Check sheet for the modelled part. Datum: model origin and axes. Units: mm. A direction names the side the tool comes from. Round coordinates to 2 decimals unless told otherwise and drop trailing zeros. Write each loop counter-clockwise with the first axis right and the second up, starting at its lowest first coordinate (ties: lowest second). Pieces come first, ordered by that corner, then holes.
Item 1: Cross-section at B-B on x = 10.75. Enter the section's corners in (y, z).
Item 2: Release check for a two-part mould opening along Y. For faces 4 (the flat face through (11, -1, 1.8)), 5 (the flat face through (0, 0, 0)), 6 (the flat face through (2, -8, 0)) record: +Y half, -Y half, draft (parallel to the pull), parting line (faces both ways), or undercut.
Item 3: Material ranges on line 1 (Y direction, x = 11.25, z = 0.2); line 2 (Y direction, x = -3, z = -0.7); line 3 (Y direction, x = 7, z = 0.6), recorded low to high.
Item 4: Tool access check on faces 1 (the flat face through (8.8, -3.3, -0.2)), 2 (the flat face through (4, -7, 1.8)), 3 (the flat face through (9, 1, 1)). Record the directions out of +Z, -Z, +X, -X, +Y, -Y that give a thin tool (end or side, any length) a straight path to the whole face; none if there is none.
Item 5: Cross-section at D-D on x = -3. Enter the section's corners in (y, z), plus the area to 4 significant figures.
Item 6: Cross-section at A-A on z = 0.8. Enter the section's corners in (x, y), plus the area to 3 significant figures.
Item 7: Cross-section at C-C on y = 0. Enter the section's corners in (x, z).
Item 8: Go/stop test with flat-tipped pins: pin 1 Ø0.5 at (y, z) = (3, -1) entering from +X; pin 2 Ø0.5 at (y, z) = (4.5, 1) entering from -X; pin 3 Ø1.5 at (x, y) = (0.5, 2) entering from +Z. Record where each tip stops, or that it passes through.
Autodesk Fusion 360 part; units mm, degrees
sketch "Main Body" plane through (0, 0, 0) normal (0, 0, 1) x (1, 0, 0)
  line L0 (9, 8) -> (-9, 8)
  line L1 (-9, 8) -> (-9, -8)
  line L2 (-9, -8) -> (9, -8)
  line L3 (9, -8) -> (9, 8)
  line L4 (9, 8) -> (-9, -8) construction
  line L5 (-9, 8) -> (9, -8) construction
  line L6 (9, 8) -> (13, 8)
  line L7 (13, 8) -> (13, -8)
  line L8 (13, -8) -> (9, -8)
  line L9 (9, -8) -> (9, 8)
  line L10 (9, 6) -> (-9, 6)
  line L11 (-9, -6) -> (9, -6)
  line L12 (2, 3.3) -> (13, 3.3)
  line L13 (13, 3.3) -> (13, 2.7)
  line L14 (13, 2.7) -> (2, 2.7)
  line L15 (2, 2.7) -> (2, 3.3)
  circle A0 centre (-3, 0) radius 0.85
  point P0 (2, 3)
  dimension "d4" = 18
  dimension "d5" = 4
  dimension "d7" = 16
  dimension "d8" = -2
  dimension "d9" = -2
  dimension "d10" = 0.6
  dimension "d11" = 7
  dimension "d12" = 3
  dimension "d26" = 1.7
  dimension "d27" = 6
extrude "Base" add sketch "Main Body" against normal blind 1.5 contours L0 L1 L3 L9 L10 | L3 L6 L7 L9 L12 | L1 L3 L9 L10 L11 L12 L14 L15 | L3 L7 L9 L12 L13 L14 | L3 L9 L12 L14 L15 | L1 L2 L3 L9 L11 | L3 L7 L8 L9 L14 | A0
extrude "Guide" add sketch "Main Body" along normal blind 1.8 contours L0 L1 L3 L9 L10 | L3 L6 L7 L9 L12 | L3 L7 L9 L12 L13 L14 | L1 L2 L3 L9 L11 | L3 L7 L8 L9 L14
extrude "Bristle Cut" cut sketch "Main Body" along normal through all and the other way through all contours L3 L7 L9 L12 L13 L14 | L3 L9 L12 L14 L15
pattern_linear "Bristle Pattern" count 3 spacing 3 along (0, -1, 0) of "Bristle Cut"
extrude "Fixing Hole" cut sketch "Main Body" against normal through all contours A0
equation "SegmentLength = 18 mm"
equation "d4 = SegmentLength"
equation "BandWidth = 12 mm"
equation "d7 = BandWidth + 4 mm"
equation "d11 = SegmentLength - 11 mm"
equation "d12 = BandWidth / NumBristles"
equation "d15 = BandThickness - 0.2 mm"
equation "d19 = NumBristles - 1"
equation "BandThickness = 2 mm"
Response values:
1. outline: (-8, -1.5) - (-3.3, -1.5) - (-3.3, 1.8) - (-8, 1.8) - close; (-2.7, -1.5) - (-0.3, -1.5) - (-0.3, 1.8) - (-2.7, 1.8) - close; (0.3, -1.5) - (2.7, -1.5) - (2.7, 1.8) - (0.3, 1.8) - close; (3.3, -1.5) - (8, -1.5) - (8, 1.8) - (3.3, 1.8) - close
2. face 4: draft
2. face 5: undercut
2. face 6: -Y half
3. line 1: y = -8 to -3.3, -2.7 to -0.3, 0.3 to 2.7, 3.3 to 8
3. line 2: y = -8 to -0.85, 0.85 to 8
3. line 3: y = -8 to -6, 6 to 8
4. face 1: +Z, -Z, +X
4. face 2: +Z, +X, -X, +Y, -Y
4. face 3: +Z, -X
5. outline: (-8, -1.5) - (-0.85, -1.5) - (-0.85, 0) - (-6, 0) - (-6, 1.8) - (-8, 1.8) - close; (0.85, -1.5) - (8, -1.5) - (8, 1.8) - (6, 1.8) - (6, 0) - (0.85, 0) - close
5. area: 28.65 mm2
6. outline: (-9, -8) - (13, -8) - (13, -3.3) - (9, -3.3) - (9, -6) - (-9, -6) - close; (-9, 6) - (9, 6) - (9, 3.3) - (13, 3.3) - (13, 8) - (-9, 8) - close; (9, -2.7) - (13, -2.7) - (13, -0.3) - (9, -0.3) - close; (9, 0.3) - (13, 0.3) - (13, 2.7) - (9, 2.7) - close
6. area: 129 mm2
7. outline: (-9, -1.5) - (-3.85, -1.5) - (-3.85, 0) - (-9, 0) - close; (-2.15, -1.5) - (2, -1.5) - (2, 0) - (-2.15, 0) - close
8. pin 1: stops at x = 2
8. pin 2: stops at x = 9
8. pin 3: stops at z = 0
